Geometry: final body of the model. Coordinates: model frame, mm. Give positions to 0.01 mm unless a question says otherwise; leave off trailing zeros. Order: outer loops, then holes, each group sorted by start corner. A loop starts at its lowest first (then second) coordinate and runs counter-clockwise, first axis right, second up. Notation, with made-up numbers: M 33,32 L 40,32 A7 ccw 40,37 Z; hole C 81,45 d11. An arc over 180 degrees is marked long. One line per item, written item: value. Start each with the question number.
```python
from build123d import *

# Parameters (mm, degrees)
SKETCH1_R           = 0.1
BOSS_EXTRUDE2_DEPTH = 0.18
FILLET1_R           = 0.5


with BuildPart() as part:
    # Sketch1 → Boss-Extrude2 (new body)
    with BuildSketch(Plane(origin=(0, 0, 0), x_dir=(1, 0, 0), z_dir=(0, 1, 0))):
        with BuildLine():
            Line((-0.4, -3.945683229), (-0.4, -1.445683229))
            ThreePointArc((-0.4, -1.445683229), (-1.5, 0), (-0.4, 1.445683229))
            Line((-0.4, 1.445683229), (-0.4, 14.554316771))
            Line((-0.4, 14.554316771), (0.4, 14.554316771))
            Line((0.4, 14.554316771), (0.4, 1.445683229))
            ThreePointArc((0.4, 1.445683229), (1.5, 0), (0.4, -1.445683229))
            Line((0.4, -1.445683229), (0.4, -3.945683229))
            Line((0.4, -3.945683229), (-0.4, -3.945683229))
        make_face()
        with Locations(Location((0, 0, 0), (0, 0, 270))):
            Circle(SKETCH1_R, mode=Mode.SUBTRACT)
    extrude(amount=BOSS_EXTRUDE2_DEPTH)

    # Fillet1
    # the kernel refuses this fillet: 0.5 mm, written as the material it takes off along each edge
    with BuildSketch(Plane(origin=(-0.4, -1.25, -14.554316771), x_dir=(0, 0, 1), z_dir=(0, 1, 0)), Plane(origin=(0.4, -1.25, -14.554316771), x_dir=(-1, 0, 0), z_dir=(0, 1, 0)), Plane(origin=(-0.4, -1.25, 3.945683229), x_dir=(1, 0, 0), z_dir=(0, 1, 0)), Plane(origin=(0.4, -1.25, 3.945683229), x_dir=(0, 0, -1), z_dir=(0, 1, 0))) as fillet1_piece_1:
        with BuildLine():
            CenterArc((FILLET1_R, FILLET1_R), FILLET1_R, 180, 90)
            Line((0, FILLET1_R), (0, 0))
            Line((0, 0), (FILLET1_R, 0))
        make_face()
    extrude(amount=2.68, mode=Mode.SUBTRACT)


solid = part.part
```
Q1. Section query B-B on z = -10. Return loops of the section in (x, y), and give its area (3 significant figures).
Q2. Section query A-A on y = 0.1. Return loops of the section in (x, z), and give its area (3 significant figures).
Q3. Section query C-C on x = 1.3. Return loops of the section in (y, z).
Q4. Ray query, line 1 along X through (y, z) = (0.1, 0); line 2 along X through (y, z) = (0.1, -4); line 3 along Z through (x, y) = (-0.45, 0.1). Return the intervals inside material, ascending. Write a range as [from, to].
Results below:
1. outline: M -0.4,0 L 0.4,0 L 0.4,0.18 L -0.4,0.18 Z
1. area: 0.144 mm2
2. outline: M -0.4,-14.05 A0.5 ccw 0,-14.54 A0.5 ccw 0.4,-14.05 L 0.4,-1.45 A1.5 ccw 0.4,1.45 L 0.4,3.45 A0.5 ccw 0,3.94 A0.5 ccw -0.4,3.45 L -0.4,1.45 A1.5 ccw -0.4,-1.45 Z; hole C 0,0 d0.2
2. area: 19.3 mm2
3. outline: M 0,-0.75 L 0.18,-0.75 L 0.18,0.75 L 0,0.75 Z
4. line 1: [-1.5, -0.1], [0.1, 1.5]
4. line 2: [-0.4, 0.4]
4. line 3: [-1.43, 1.43]
